```python
from build123d import *

# Parameters (mm, degrees)
SKETCH1_W           = 35
SKETCH1_H           = 60
BOSS_EXTRUDE1_DEPTH = 3
BOSS_EXTRUDE2_DEPTH = 25
CUT_EXTRUDE1_DEPTH  = 1
CHAMFER1_SIZE       = 11.547005384
CHAMFER1_SIZE_2     = 20


with BuildPart() as part:
    # Sketch1 → Boss-Extrude1 (new body)
    with BuildSketch(Plane(origin=(0, 0, 0), x_dir=(1, 0, 0), z_dir=(0, 1, 0))):
        Rectangle(SKETCH1_W, SKETCH1_H)
    extrude(amount=BOSS_EXTRUDE1_DEPTH)

    # Sketch2 → Boss-Extrude2 (add)
    with BuildSketch(Plane(origin=(0, 3, 0), x_dir=(1, 0, 0), z_dir=(0, 1, 0))):
        with BuildLine():
            Line((-2.598076211, 13), (-15.155444566, -8.75))
            Line((-15.155444566, -8.75), (15.155444566, -8.75))
            Line((15.155444566, -8.75), (2.598076211, 13))
            ThreePointArc((2.598076211, 13), (0, 14.5), (-2.598076211, 13))
        make_face()
    extrude(amount=BOSS_EXTRUDE2_DEPTH)

    # Sketch3 → Cut-Extrude1 (cut)
    with BuildSketch(Plane(origin=(0, 3, 0), x_dir=(1, 0, 0), z_dir=(0, 1, 0))):
        with BuildLine():
            Line((-6.495190528, -3.75), (0, 7.5))
            Line((0, 7.5), (6.495190528, -3.75))
            Line((6.495190528, -3.75), (9.381941874, -8.75))
            Line((9.381941874, -8.75), (15.155444566, -8.75))
            Line((15.155444566, -8.75), (2.598076211, 13))
            ThreePointArc((2.598076211, 13), (0, 14.5), (-2.598076211, 13))
            Line((-2.598076211, 13), (-15.155444566, -8.75))
            Line((-15.155444566, -8.75), (-9.381941874, -8.75))
            Line((-9.381941874, -8.75), (-6.495190528, -3.75))
        make_face()
    extrude(amount=CUT_EXTRUDE1_DEPTH, mode=Mode.SUBTRACT)

    # Chamfer1
    # the kernel refuses this chamfer: 20, 11.547005384 mm, written as the material it takes off along each edge
    with BuildSketch(Plane(origin=(41.026302113, 4, 53.559639706), x_dir=(-0.8645728572665647, -0.057893862402670825, 0.4991613718769001), z_dir=(-0.5000000000000038, 0, -0.8660254037844365))) as chamfer1_piece_1_section:
        Polygon((CHAMFER1_SIZE * 0.998322743736, CHAMFER1_SIZE * 0.0578938624016), (-CHAMFER1_SIZE_2 * 0.0578938624027, CHAMFER1_SIZE_2 * 0.998322743754), (0, 0), align=None)
    chamfer1_piece_1 = extrude(amount=128.598166896, mode=Mode.PRIVATE)
    chamfer1_piece_1 = split(chamfer1_piece_1, bisect_by=Plane(origin=(4.860727158, 12.114805615, 0.9190264), z_dir=(0.8660254037844364, 0, -0.500000000000004)), keep=Keep.TOP, mode=Mode.PRIVATE)
    add(chamfer1_piece_1, mode=Mode.SUBTRACT)
    with BuildSketch(Plane(origin=(41.026302113, 4, 53.559639706), x_dir=(-0.8645728572665647, -0.057893862402670825, 0.4991613718769001), z_dir=(-0.5000000000000038, 0, -0.8660254037844365))) as chamfer1_piece_2_section:
        Polygon((CHAMFER1_SIZE * 0.998322743736, CHAMFER1_SIZE * 0.0578938624016), (-CHAMFER1_SIZE_2 * 0.0578938624027, CHAMFER1_SIZE_2 * 0.998322743754), (0, 0), align=None)
    chamfer1_piece_2 = extrude(amount=128.598166896, mode=Mode.PRIVATE)
    chamfer1_piece_2 = split(chamfer1_piece_2, bisect_by=Plane(origin=(-0.762291107, 7.498768365, -6.179673073), z_dir=(-0.8660254037844386, 0, -0.5000000000000001)), keep=Keep.TOP, mode=Mode.PRIVATE)
    add(chamfer1_piece_2, mode=Mode.SUBTRACT)
    with BuildSketch(Plane(origin=(23.272781335, 4, -57.809639706), x_dir=(0.864572857266568, -0.05789386240267081, 0.49916137187689447), z_dir=(-0.49999999999999817, 0, 0.8660254037844398))) as chamfer1_piece_3_section:
        Polygon((CHAMFER1_SIZE * 0.998322743736, CHAMFER1_SIZE * 0.0578938624016), (-CHAMFER1_SIZE_2 * 0.0578938624027, CHAMFER1_SIZE_2 * 0.998322743754), (0, 0), align=None)
    chamfer1_piece_3 = extrude(amount=128.598166896, mode=Mode.PRIVATE)
    chamfer1_piece_3 = split(chamfer1_piece_3, bisect_by=Plane(origin=(0.762291107, 7.498768365, -6.179673073), z_dir=(0.8660254037844364, 0, -0.500000000000004)), keep=Keep.TOP, mode=Mode.PRIVATE)
    add(chamfer1_piece_3, mode=Mode.SUBTRACT)
    with BuildSketch(Plane(origin=(23.272781335, 4, -57.809639706), x_dir=(0.864572857266568, -0.05789386240267081, 0.49916137187689447), z_dir=(-0.49999999999999817, 0, 0.8660254037844398))) as chamfer1_piece_4_section:
        Polygon((CHAMFER1_SIZE * 0.998322743736, CHAMFER1_SIZE * 0.0578938624016), (-CHAMFER1_SIZE_2 * 0.0578938624027, CHAMFER1_SIZE_2 * 0.998322743754), (0, 0), align=None)
    chamfer1_piece_4 = extrude(amount=128.598166896, mode=Mode.PRIVATE)
    chamfer1_piece_4 = split(chamfer1_piece_4, bisect_by=Plane(origin=(-4.860727158, 12.114805615, 0.9190264), z_dir=(-0.8660254037844386, 0, -0.5000000000000001)), keep=Keep.TOP, mode=Mode.PRIVATE)
    add(chamfer1_piece_4, mode=Mode.SUBTRACT)


solid = part.part
```
Work out the finished part from the listing and answer in its coordinate system (mm). A direction names the side the tool comes from. Round coordinates to 2 decimals unless told otherwise and drop trailing zeros. Loops run counter-clockwise (first coordinate to the right, second up) from the corner with the lowest first, then second, coordinate; pieces in that order, holes last. Notation, with made-up numbers: (-30, 24) -> (-7, 24) arc R21 ccw to (-7, 58) -> close; hole circle Ø3 at (77.5, 41.25). An arc over 180 degrees is marked (long way). Write each question's results on one line, items separated by ' | '. Start each with the question number.
1. Section A-A (x = 11) is taken. Determine the outline of the cut face in (y, z), plus the area to 3 significant figures.
2. Section B-B (z = -11.5) is taken. Determine the outline of the cut face in (x, y).
3. Given pin 1 Ø10 at (y, z) = (15, -11) entering from +X; pin 2 Ø2 at (y, z) = (12, 5.5) entering from -X; pin 3 Ø10 at (x, y) = (6.5, 13) entering from +Z; pin 4 Ø4 at (y, z) = (5.5, 18.5) entering from -X, each flat-ended and moving along its own axis, determine where each tip first touches the part or whether it passes through.
4. For a pull along Y with two mould halves and no side action, classify faces 1 (the face through (-5.9, 19.6, -2.2)), 2 (the face through (0, 0, 0)), 3 (the face through (17.5, 1, 0)) as +Y half, -Y half, draft (parallel to the pull), parting line (faces both ways), or undercut.
5. Find the intervals of material crossed by probe 1 along Z at (x, y) = (6.5, 8.5); probe 2 along Y at (x, z) = (-10.5, 10); probe 3 along Y at (x, z) = (-1.5, -14), in increasing order. Write a range as from..to.
6. Section D-D (y = 5.25) is taken. Determine the outline of the cut face in (x, z), plus the area to 3 significant figures.
7. A tool of negligible diameter and unlimited length cuts with its end or side. For faces 4 (the face through (0, 25.4, -14.5)), 5 (the face through (0, 18, 8.75)), 6 (the face through (-4, 3, -7)), 7 (the face through (6.13, 19.61, -1.81)), from which of +Z, -Z, +X, -X, +Y, -Y can it reach the whole face along a straight path? Write none if from no direction.
8. Section C-C (x = -5.5) is taken. Determine the outline of the cut face in (y, z).
Evaluation:
1) outline: (0, -30) -> (3, -30) -> (3, 30) -> (0, 30) -> close; (17.77, 8.75) -> (24, 1.55) -> (28, 1.55) -> (28, 8.75) -> close | area: 231 mm2
2) outline: (-17.5, 0) -> (17.5, 0) -> (17.5, 3) -> (-17.5, 3) -> close; (-3.46, 24) -> (0, 18.8) -> (3.46, 24) -> (3.46, 28) -> (-3.46, 28) -> close
3) pin 1: stops at x = 2.16 | pin 2: stops at x = -8.08 | pin 3: stops at z = 8.75 | pin 4: passes through
4) face 1: undercut | face 2: -Y half | face 3: draft
5) probe 1: z = 3.76..8.75 | probe 2: y = 0..3 | probe 3: y = 0..3, 23.22..28
6) outline: (-9.38, 8.75) -> (0, -7.5) -> (9.38, 8.75) -> close | area: 152 mm2
7) face 4: -Z, +Y | face 5: +Z, +X, -X, +Y | face 6: none | face 7: -Z, +X
8) outline: (0, -30) -> (3, -30) -> (3, 2.03) -> (15.34, 2.03) -> (24, -7.97) -> (28, -7.97) -> (28, 8.75) -> (3, 8.75) -> (3, 30) -> (0, 30) -> close
